from build123d import *

# Parameters (mm, degrees)
F0_W     = 90
F0_H     = 90
F0_R     = 3.25
F1_DEPTH = 10
F3_DEPTH = 2
F5_DEPTH = 10.001


with BuildPart() as f1:
    # F0 (on Front) → F1 (new body)
    with BuildSketch(Plane.XZ):
        Rectangle(F0_W, F0_H)
        with Locations((-34.8, -34.8)):
            Circle(F0_R, mode=Mode.SUBTRACT)
        with Locations((34.8, -34.8)):
            Circle(F0_R, mode=Mode.SUBTRACT)
        with Locations((-34.8, 34.8)):
            Circle(F0_R, mode=Mode.SUBTRACT)
        with Locations((34.8, 34.8)):
            Circle(F0_R, mode=Mode.SUBTRACT)
    extrude(amount=F1_DEPTH)

    # F2 (on Front) → F3 (cut)
    with BuildSketch(Plane.XZ):
        with BuildLine():
            ThreePointArc((36.5, 32.5), (35.328427, 35.328427), (32.5, 36.5))
            Line((32.5, 36.5), (-32.5, 36.5))
            ThreePointArc((-32.5, 36.5), (-35.328427, 35.328427), (-36.5, 32.5))
            Line((-36.5, 32.5), (-36.5, -32.5))
            ThreePointArc((-36.5, -32.5), (-35.328427, -35.328427), (-32.5, -36.5))
            Line((-32.5, -36.5), (32.5, -36.5))
            ThreePointArc((32.5, -36.5), (35.328427, -35.328427), (36.5, -32.5))
            Line((36.5, -32.5), (36.5, 32.5))
        make_face()
    extrude(amount=F3_DEPTH, mode=Mode.SUBTRACT)

    # F4 (on Front) → F5 (cut, through all)
    with BuildSketch(Plane.XZ):
        with BuildLine():
            ThreePointArc((22.5, 16.5), (20.742641, 20.742641), (16.5, 22.5))
            Line((16.5, 22.5), (-16.5, 22.5))
            ThreePointArc((-16.5, 22.5), (-20.742641, 20.742641), (-22.5, 16.5))
            Line((-22.5, 16.5), (-22.5, -16.5))
            ThreePointArc((-22.5, -16.5), (-20.742641, -20.742641), (-16.5, -22.5))
            Line((-16.5, -22.5), (16.5, -22.5))
            ThreePointArc((16.5, -22.5), (20.742641, -20.742641), (22.5, -16.5))
            Line((22.5, -16.5), (22.5, 16.5))
        make_face()
    extrude(amount=F5_DEPTH, mode=Mode.SUBTRACT)


solid = f1.part
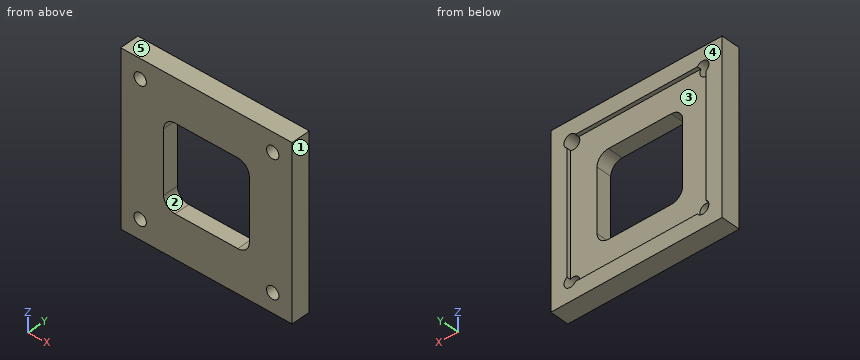
Work out the finished part from the listing and answer in its coordinate system (mm). Face numbers are marked on the shaded views. A direction names the side the tool comes from. Give positions to 0.01 mm unless a question says otherwise; leave off trailing zeros. Loops run counter-clockwise (first coordinate to the right, second up) from the corner with the lowest first, then second, coordinate; pieces in that order, holes last. Notation, with made-up numbers: (84.25, -29) -> (97.25, -29) arc R11 cw to (97.25, -12) -> close; hole circle Ø7 at (21.25, 81.5). An arc over 180 degrees is marked (long way). Use a Markdown table: item, result. Add a question column.
1) Each of these flat-tipped pins is pushed along its axis until it touches: P1, Ø7.5, axis at x = -34.8, z = -34.8, coming from the -Y side; P2, Ø10, axis at x = 15.5, z = 21, coming from the +Y side. Where does it stop, or does it pass through?
2) The part is cut by section C-C, the plane y = -3.5. Determine the outline of the cut face in (x, z).
3) The part is cut by section A-A, the plane x = 7. Determine the outline of the cut face in (y, z), plus the area to 3 significant figures.
4) The part is cut by section B-B, the plane z = 34.8. Determine the outline of the cut face in (x, y).
5) For a pull along Z with two mould halves and no side action, classify the marked faces 3, 4 and 5 as +Z half, -Z half, draft (parallel to the pull), parting line (faces both ways), or undercut.
6) Which of the six approach directions +Z, -Z, +X, -X, +Y, -Y give full straight-line access (tool end or side, diameter ignored) to the marked faces 1 and 2?
7) Consider line 1 along Z through (x, y) = (34.8, -6.5); line 2 along Z through (x, y) = (20, -0.75). Determine where each line is inside the solid, lowest interval first.
8) The part is cut by section D-D, the plane x = -34.8. Determine the outline of the cut face in (y, z).
Reported:
| question | item | result |
|---|---|---|
| 1 | P1 | stops at y = -10 |
| 1 | P2 | stops at y = -2 |
| 2 | outline | (-45, -45) -> (45, -45) -> (45, 45) -> (-45, 45) -> close; hole circle Ø6.5 at (-34.8, -34.8); hole circle Ø6.5 at (-34.8, 34.8); hole (-22.5, -16.5) arc R6 ccw to (-16.5, -22.5) -> (16.5, -22.5) arc R6 ccw to (22.5, -16.5) -> (22.5, 16.5) arc R6 ccw to (16.5, 22.5) -> (-16.5, 22.5) arc R6 ccw to (-22.5, 16.5) -> close; hole circle Ø6.5 at (34.8, -34.8); hole circle Ø6.5 at (34.8, 34.8) |
| 3 | outline | (-10, -45) -> (0, -45) -> (0, -36.5) -> (-2, -36.5) -> (-2, -22.5) -> (-10, -22.5) -> close; (-10, 22.5) -> (-2, 22.5) -> (-2, 36.5) -> (0, 36.5) -> (0, 45) -> (-10, 45) -> close |
| 3 | area | 394 mm^2 |
| 4 | outline | (-45, -10) -> (-38.05, -10) -> (-38.05, 0) -> (-45, 0) -> close; (-31.55, -10) -> (31.55, -10) -> (31.55, -2) -> (-31.55, -2) -> close; (38.05, -10) -> (45, -10) -> (45, 0) -> (38.05, 0) -> close |
| 5 | face 3 | undercut |
| 5 | face 4 | draft |
| 5 | face 5 | +Z half |
| 6 | face 1 | +Z, -Z, +X, +Y, -Y |
| 6 | face 2 | +Y, -Y |
| 7 | line 1 | z = -45 to -38.05, -31.55 to 31.55, 38.05 to 45 |
| 7 | line 2 | z = -45 to -36.5, 36.5 to 45 |
| 8 | outline | (-10, -45) -> (0, -45) -> (0, -38.05) -> (-10, -38.05) -> close; (-10, -31.55) -> (-2, -31.55) -> (-2, 31.55) -> (-10, 31.55) -> close; (-10, 38.05) -> (0, 38.05) -> (0, 45) -> (-10, 45) -> close |
